Model file for the job. Use its own axes, mm. A direction names the side the tool comes from. Round coordinates to 2 decimals unless told otherwise and drop trailing zeros. Order: outer loops, then holes, each group sorted by start corner. A loop starts at its lowest first (then second) coordinate and runs counter-clockwise, first axis right, second up. Notation, with made-up numbers: M 29.5,74.5 L 37.5,74.5 A18 ccw 37.5,79.5 Z; hole C -16.5,26 d4. An arc over 180 degrees is marked long. Return JSON: item names as keys, results as strings. Group by question number.
Item 1: Probe line 1 along X through (y, z) = (0.4, 23); line 2 along X through (y, z) = (2.25, 21); line 3 along X through (y, z) = (0.85, -20.5). List the from-to ranges inside material, lowest first.
Item 2: Pull direction Z, two halves, no side cores. Call faces 4 (the face through (-9.805, 1.257, -22.743)), 5 (the face through (-22.62, 1.26, 10)), 6 (the face through (-8.28, 1.26, 23.34)): pulls with the +Z half, pulls with the -Z half, needs draft (parallel to the pull), parting line crosses it, or undercut.
Item 3: Slice it at B-B on z = 11.75. Write the cut outline in (x, y), then the cut area to 3 significant figures.
Item 4: Pin check, flat tips, straight feed: pin 1 Ø1 at (y, z) = (1.5, -4.5) entering from -X; pin 2 Ø8 at (x, z) = (-5.5, 1.5) entering from -Y. Stop position of each tip, or through.
Item 5: Slice it at A-A on z = 0. Write the cut outline in (x, y).
Item 6: Which spindle directions (+Z, -Z, +X, -X, +Y, -Y) get a long thin tool onto all of the face, cutting with end or side? Do faces 1 (the face through (24.7, 1.3, 0.8)), 2 (the face through (-19.99, 1.26, 14.62)), 3 (the face through (23.859, 1.257, -6.516)). Say none if no direction does.
from build123d import *

# Parameters (mm, degrees)
SKETCH1_R               = 3
BOSS_EXTRUDE1_DEPTH     = 2.55
SKETCH2_R               = 10
CUT_EXTRUDE1_DEPTH      = 4
CUT_EXTRUDE1_DEPTH_BACK = 4


with BuildPart() as part:
    # Sketch1 → Boss-Extrude1 (new body)
    with BuildSketch(Plane(origin=(0, 0, 0), x_dir=(1, 0, 0), z_dir=(0, 1, 0))):
        with BuildLine():
            ThreePointArc((-2.496460827, 23.367021277), (0, 21), (2.496460827, 23.367021277))
            ThreePointArc((2.496460827, 23.367021277), (2.658416444, 24.60643544), (3.524555237, 25.507646116))
            ThreePointArc((3.524555237, 25.507646116), (3.837838354, 25.462393775), (4.150541543, 25.413293862))
            ThreePointArc((4.150541543, 25.413293862), (4.712563709, 24.296822557), (4.502000355, 23.064734831))
            ThreePointArc((4.502000355, 23.064734831), (6.189858663, 20.067028922), (9.273100509, 21.593045338))
            ThreePointArc((9.273100509, 21.593045338), (9.79318463, 22.729658551), (10.886479817, 23.335532074))
            ThreePointArc((10.886479817, 23.335532074), (11.172506282, 23.199948348), (11.456844492, 23.060858923))
            ThreePointArc((11.456844492, 23.060858923), (11.664811896, 21.828330364), (11.100439049, 20.713045477))
            ThreePointArc((11.100439049, 20.713045477), (11.829721219, 17.351014261), (15.225784516, 17.900432561))
            ThreePointArc((15.225784516, 17.900432561), (16.057785385, 18.833251753), (17.28109289, 19.089953602))
            ThreePointArc((17.28109289, 19.089953602), (17.514447998, 18.8760857), (17.745156531, 18.659365469))
            ThreePointArc((17.745156531, 18.659365469), (17.580590356, 17.420295227), (16.712555019, 16.520911135))
            ThreePointArc((16.712555019, 16.520911135), (16.418461132, 13.093285839), (19.825590752, 12.617287797))
            ThreePointArc((19.825590752, 12.617287797), (20.895581441, 13.263427887), (22.140205024, 13.148148977))
            ThreePointArc((22.140205024, 13.148148977), (22.300154147, 12.875), (22.456733538, 12.599905507))
            ThreePointArc((22.456733538, 12.599905507), (21.934256212, 11.464390411), (20.839687135, 10.860821338))
            ThreePointArc((20.839687135, 10.860821338), (19.548348722, 7.672161512), (22.663806246, 6.213041642))
            ThreePointArc((22.663806246, 6.213041642), (23.876713386, 6.515090249), (25.03206278, 6.038073615))
            ThreePointArc((25.03206278, 6.038073615), (25.104393739, 5.729914049), (25.172931221, 5.420888647))
            ThreePointArc((25.172931221, 5.420888647), (24.338967146, 4.489824196), (23.115121595, 4.235699903))
            ThreePointArc((23.115121595, 4.235699903), (20.941279741, 1.569331965), (23.488243097, -0.743260529))
            ThreePointArc((23.488243097, -0.743260529), (24.736294566, -0.812141749), (25.699711907, -1.608511084))
            ThreePointArc((25.699711907, -1.608511084), (25.677997777, -1.92429991), (25.652403496, -2.239797958))
            ThreePointArc((25.652403496, -2.239797958), (24.58105404, -2.883682602), (23.336676062, -2.765782057))
            ThreePointArc((23.336676062, -2.765782057), (20.473486156, -4.672939613), (22.225646472, -7.63352074))
            ThreePointArc((22.225646472, -7.63352074), (23.39794742, -8.067211389), (24.083828849, -9.112172516))
            ThreePointArc((24.083828849, -9.112172516), (23.969999028, -9.407531377), (23.852547146, -9.701468686))
            ThreePointArc((23.852547146, -9.701468686), (22.63900641, -10.000961546), (21.48466445, -9.521512143))
            ThreePointArc((21.48466445, -9.521512143), (18.186533479, -10.5), (18.988203623, -13.845509134))
            ThreePointArc((18.988203623, -13.845509134), (19.980589966, -14.605473895), (20.327991909, -15.80617743))
            ThreePointArc((20.327991909, -15.80617743), (20.132160674, -16.054862398), (19.933287307, -16.301121346))
            ThreePointArc((19.933287307, -16.301121346), (18.685383711, -16.229611167), (17.723646117, -15.431214091))
            ThreePointArc((17.723646117, -15.431214091), (14.283627493, -15.394089308), (14.063575553, -18.827263281))
            ThreePointArc((14.063575553, -18.827263281), (14.78786941, -19.845975949), (14.765923679, -21.095734116))
            ThreePointArc((14.765923679, -21.095734116), (14.505491495, -21.275648439), (14.242867415, -21.452347839))
            ThreePointArc((14.242867415, -21.452347839), (13.071482669, -21.016188615), (12.387804048, -19.969784948))
            ThreePointArc((12.387804048, -19.969784948), (9.111558521, -18.920346226), (7.889337079, -22.136132464))
            ThreePointArc((7.889337079, -22.136132464), (8.281181761, -23.323075949), (7.891838331, -24.510842249))
            ThreePointArc((7.891838331, -24.510842249), (7.589945741, -24.605999749), (7.286906249, -24.697439084))
            ThreePointArc((7.286906249, -24.697439084), (6.29612303, -23.935385475), (5.951251227, -22.733952776))
            ThreePointArc((5.951251227, -22.733952776), (3.12988759, -20.765447351), (1.014096383, -23.478109134))
            ThreePointArc((1.014096383, -23.478109134), (1.038674771, -24.727818298), (0.316528515, -25.748054484))
            ThreePointArc((0.316528515, -25.748054484), (0, -25.75), (-0.316528515, -25.748054484))
            ThreePointArc((-0.316528515, -25.748054484), (-1.038674771, -24.727818298), (-1.014096383, -23.478109134))
            ThreePointArc((-1.014096383, -23.478109134), (-3.12988759, -20.765447351), (-5.951251227, -22.733952776))
            ThreePointArc((-5.951251227, -22.733952776), (-6.29612303, -23.935385475), (-7.286906249, -24.697439084))
            ThreePointArc((-7.286906249, -24.697439084), (-7.589945741, -24.605999749), (-7.891838331, -24.510842249))
            ThreePointArc((-7.891838331, -24.510842249), (-8.281181761, -23.323075949), (-7.889337079, -22.136132464))
            ThreePointArc((-7.889337079, -22.136132464), (-9.111558521, -18.920346226), (-12.387804048, -19.969784948))
            ThreePointArc((-12.387804048, -19.969784948), (-13.071482669, -21.016188615), (-14.242867415, -21.452347839))
            ThreePointArc((-14.242867415, -21.452347839), (-14.505491495, -21.275648439), (-14.765923679, -21.095734116))
            ThreePointArc((-14.765923679, -21.095734116), (-14.78786941, -19.845975949), (-14.063575553, -18.827263281))
            ThreePointArc((-14.063575553, -18.827263281), (-14.283627493, -15.394089308), (-17.723646117, -15.431214091))
            ThreePointArc((-17.723646117, -15.431214091), (-18.685383711, -16.229611167), (-19.933287307, -16.301121346))
            ThreePointArc((-19.933287307, -16.301121346), (-20.132160674, -16.054862398), (-20.327991909, -15.80617743))
            ThreePointArc((-20.327991909, -15.80617743), (-19.980589966, -14.605473895), (-18.988203623, -13.845509134))
            ThreePointArc((-18.988203623, -13.845509134), (-18.186533479, -10.5), (-21.48466445, -9.521512143))
            ThreePointArc((-21.48466445, -9.521512143), (-22.63900641, -10.000961546), (-23.852547146, -9.701468686))
            ThreePointArc((-23.852547146, -9.701468686), (-23.969999028, -9.407531377), (-24.083828849, -9.112172516))
            ThreePointArc((-24.083828849, -9.112172516), (-23.39794742, -8.067211389), (-22.225646472, -7.63352074))
            ThreePointArc((-22.225646472, -7.63352074), (-20.473486156, -4.672939613), (-23.336676062, -2.765782057))
            ThreePointArc((-23.336676062, -2.765782057), (-24.58105404, -2.883682602), (-25.652403496, -2.239797958))
            ThreePointArc((-25.652403496, -2.239797958), (-25.677997777, -1.92429991), (-25.699711907, -1.608511084))
            ThreePointArc((-25.699711907, -1.608511084), (-24.736294566, -0.812141749), (-23.488243097, -0.743260529))
            ThreePointArc((-23.488243097, -0.743260529), (-20.941279741, 1.569331965), (-23.115121595, 4.235699903))
            ThreePointArc((-23.115121595, 4.235699903), (-24.338967146, 4.489824196), (-25.172931221, 5.420888647))
            ThreePointArc((-25.172931221, 5.420888647), (-25.104393739, 5.729914049), (-25.03206278, 6.038073615))
            ThreePointArc((-25.03206278, 6.038073615), (-23.876713386, 6.515090249), (-22.663806246, 6.213041642))
            ThreePointArc((-22.663806246, 6.213041642), (-19.548348722, 7.672161512), (-20.839687135, 10.860821338))
            ThreePointArc((-20.839687135, 10.860821338), (-21.934256212, 11.464390411), (-22.456733538, 12.599905507))
            ThreePointArc((-22.456733538, 12.599905507), (-22.300154147, 12.875), (-22.140205024, 13.148148977))
            ThreePointArc((-22.140205024, 13.148148977), (-20.895581441, 13.263427887), (-19.825590752, 12.617287797))
            ThreePointArc((-19.825590752, 12.617287797), (-16.418461132, 13.093285839), (-16.712555019, 16.520911135))
            ThreePointArc((-16.712555019, 16.520911135), (-17.580590356, 17.420295227), (-17.745156531, 18.659365469))
            ThreePointArc((-17.745156531, 18.659365469), (-17.514447998, 18.8760857), (-17.28109289, 19.089953602))
            ThreePointArc((-17.28109289, 19.089953602), (-16.057785385, 18.833251753), (-15.225784516, 17.900432561))
            ThreePointArc((-15.225784516, 17.900432561), (-11.829721219, 17.351014261), (-11.100439049, 20.713045477))
            ThreePointArc((-11.100439049, 20.713045477), (-11.664811896, 21.828330364), (-11.456844492, 23.060858923))
            ThreePointArc((-11.456844492, 23.060858923), (-11.172506282, 23.199948348), (-10.886479817, 23.335532074))
            ThreePointArc((-10.886479817, 23.335532074), (-9.79318463, 22.729658551), (-9.273100509, 21.593045338))
            ThreePointArc((-9.273100509, 21.593045338), (-6.189858663, 20.067028922), (-4.502000355, 23.064734831))
            ThreePointArc((-4.502000355, 23.064734831), (-4.712563709, 24.296822557), (-4.150541543, 25.413293862))
            ThreePointArc((-4.150541543, 25.413293862), (-3.837838354, 25.462393775), (-3.524555237, 25.507646116))
            ThreePointArc((-3.524555237, 25.507646116), (-2.658416444, 24.60643544), (-2.496460827, 23.367021277))
        make_face()
        with Locations((-6.5, 0)):
            Circle(SKETCH1_R, mode=Mode.SUBTRACT)
        with Locations((0, 7)):
            Circle(SKETCH1_R, mode=Mode.SUBTRACT)
        with Locations((7, 0)):
            Circle(SKETCH1_R, mode=Mode.SUBTRACT)
        with Locations((0, -7)):
            Circle(SKETCH1_R, mode=Mode.SUBTRACT)
    extrude(amount=BOSS_EXTRUDE1_DEPTH)

    # Sketch2 → Cut-Extrude1 (cut, two sides)
    with BuildSketch(Plane(origin=(0, 1.275, 0), x_dir=(1, 0, 0), z_dir=(0, 1, 0))) as cut_extrude1_sk:
        Circle(SKETCH2_R)
    extrude(amount=CUT_EXTRUDE1_DEPTH, mode=Mode.SUBTRACT)
    extrude(cut_extrude1_sk.sketch, amount=-CUT_EXTRUDE1_DEPTH_BACK, mode=Mode.SUBTRACT)


solid = part.part
Output values:
{
 "1": {"line 1": "-8.25 to -5.96, -1.01 to 1.01, 5.96 to 8.25", "line 2": "-14.8 to -13.05, -7.7 to -4.62, -2.39 to 2.39, 4.62 to 7.7, 13.05 to 14.8", "line 3": "-10.98 to -8.48, -5.37 to 5.37, 8.48 to 10.98"},
 "2": {"face 4": "pulls with the -Z half", "face 5": "pulls with the +Z half", "face 6": "undercut"},
 "3": {"outline": "M -17.85,0 L 17.85,0 L 17.85,2.55 L -17.85,2.55 Z", "area": "91.0 mm²"},
 "4": {"pin 1": "x = -24.92", "pin 2": "through"},
 "5": {"outline": "M -21.65,0 L -10,0 L -10,2.55 L -21.65,2.55 Z; M 10,0 L 21.65,0 L 21.65,2.55 L 10,2.55 Z"},
 "6": {"face 1": "+Y, -Y", "face 2": "-X, +Y, -Y", "face 3": "-Z, +Y, -Y"}
}
